```python
from build123d import *

# Parameters (mm, degrees)
F0_W     = 76
F0_H     = 42
F1_DEPTH = 45
F2_R     = 3
F3_T     = -2
F4_R     = 12.11184
F5_DEPTH = 25


with BuildPart() as f1:
    # F0 (on Top) → F1 (new body)
    with BuildSketch(Plane.XY):
        with Locations((7.606018, -2.175814)):
            Rectangle(F0_W, F0_H)
    extrude(amount=F1_DEPTH)

    # F2
    f2_edges = [f1.edges().sort_by_distance(p)[0] for p in [
        (-30.393982, -23.175814, 22.5),
        (-30.393982, 18.824186, 22.5),
        (45.606018, -23.175814, 22.5),
        (45.606018, 18.824186, 22.5),
    ]]
    fillet(f2_edges, radius=F2_R)

    # F3
    f3_openings = [f1.faces().sort_by_distance(p)[0] for p in [
        (7.606018, -2.175814, 45),
    ]]
    offset(amount=F3_T, openings=f3_openings)

    # F4 (on face) → F5 (cut)
    with BuildSketch(Plane.XY.offset(2)):
        with Locations((7.606018, -2.175814)):
            Circle(F4_R)
    extrude(amount=-F5_DEPTH, mode=Mode.SUBTRACT)


solid = f1.part
```
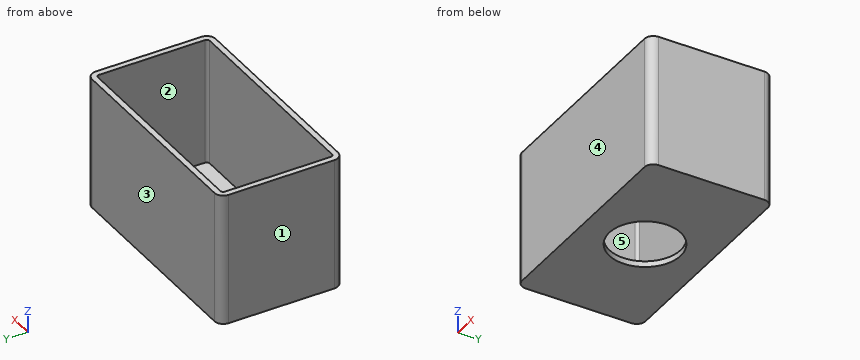
Geometry: final body of the model. Coordinates: model frame, mm. Face numbers are marked on the shaded views. A direction names the side the tool comes from. Round coordinates to 2 decimals unless told otherwise and drop trailing zeros. Write each loop counter-clockwise with the first axis right and the second up, starting at its lowest first coordinate (ties: lowest second). Pieces come first, ordered by that corner, then holes. Notation, with made-up numbers: M -33.5,-16.5 L -11.5,-16.5 A36 ccw -11.5,19.5 Z; hole C 0.25,-33 d7. An arc over 180 degrees is marked long. Answer in a Markdown table with one row per item. Add a question column.
(1) Cut plane C-C, the plane z = 6.5. Return the cut outline in (x, y), then the cut area to 3 significant figures.
(2) Reachability of the marked faces 4 and 5 from +Z, -Z, +X, -X, +Y, -Y: full face, straight path, thin tool, end or side. Return the list, or none.
(3) Contact query for flat-ended pins moving along their axis: pin 1 (5 mm diameter, centred on x = 26.5, y = -17.5, fed in from -Z); pin 2 (1.5 mm diameter, centred on x = -11.5, y = 6, fed in from +Z). Output: stop coordinate, or through.
(4) Cut plane A-A, the plane y = 5.5. Return the cut outline in (x, z), then the cut area to 3 significant figures.
(5) Draft query along X for the marked faces 1, 2 and 3. Return one class per face: pulls with the +X half, pulls with the -X half, needs draft (parallel to the pull), parting line crosses it, or undercut.
(6) Cut plane B-B, the plane x = 41. Return the cut outline in (y, z), then the cut area to 3 significant figures.
(7) Ray query, L1, parallel to X at y = 0.5, z = 22; L2, parallel to Y at x = 36, z = 37.5; L3, parallel to Z at x = -4, y = -8. Return the intervals inside material, ascending.
(8) Cut plane D-D, the plane y = 12. Return the cut outline in (x, z).
Established:
| question | item | result |
|---|---|---|
| 1 | outline | M -30.39,-20.18 A3 ccw -27.39,-23.18 L 42.61,-23.18 A3 ccw 45.61,-20.18 L 45.61,15.82 A3 ccw 42.61,18.82 L -27.39,18.82 A3 ccw -30.39,15.82 Z; hole M -28.39,-20.18 A1 ccw -27.39,-21.18 L 42.61,-21.18 A1 ccw 43.61,-20.18 L 43.61,15.82 A1 ccw 42.61,16.82 L -27.39,16.82 A1 ccw -28.39,15.82 Z |
| 1 | area | 449 mm² |
| 2 | face 4 | +Z, -Z, +X, -X, -Y |
| 2 | face 5 | +Z |
| 3 | pin 1 | z = 0 |
| 3 | pin 2 | z = 2 |
| 4 | outline | M -30.39,0 L -1.76,0 L -1.76,2 L -28.39,2 L -28.39,45 L -30.39,45 Z; M 16.98,0 L 45.61,0 L 45.61,45 L 43.61,45 L 43.61,2 L 16.98,2 Z |
| 4 | area | 287 mm² |
| 5 | face 1 | pulls with the -X half |
| 5 | face 2 | undercut |
| 5 | face 3 | needs draft |
| 6 | outline | M -23.18,0 L 18.82,0 L 18.82,45 L 16.82,45 L 16.82,2 L -21.18,2 L -21.18,45 L -23.18,45 Z |
| 6 | area | 256 mm² |
| 7 | L1 | -30.39 to -28.39, 43.61 to 45.61 |
| 7 | L2 | -23.18 to -21.18, 16.82 to 18.82 |
| 7 | L3 | 0 to 2 |
| 8 | outline | M -30.39,0 L 45.61,0 L 45.61,45 L 43.61,45 L 43.61,2 L -28.39,2 L -28.39,45 L -30.39,45 Z |
